Here's how the part is built. I have some questions about the finished solid (model axes, mm). A direction names the side the tool comes from. Round coordinates to 2 decimals unless told otherwise and drop trailing zeros. Order: outer loops, then holes, each group sorted by start corner. A loop starts at its lowest first (then second) coordinate and runs counter-clockwise, first axis right, second up.
Autodesk Inventor part; units mm, degrees
ref_plane "YZ Plane" through (0, 0, 0) normal (1, 0, 0) x (0, 1, 0)
ref_plane "XZ Plane" through (0, 0, 0) normal (0, 1, 0) x (-1, 0, 0)
ref_plane "XY Plane" through (0, 0, 0) normal (0, 0, 1) x (1, 0, 0)
sketch "Sketch1" plane through (0, 0, 0) normal (0, 1, 0) x (-1, 0, 0)
  line L0 (0, 9.8) -> (8.487, 4.9)
  line L1 (8.487, 4.9) -> (8.487, -4.9)
  line L2 (8.487, -4.9) -> (0, -9.8)
  line L3 (0, -9.8) -> (-8.487, -4.9)
  line L4 (-8.487, -4.9) -> (-8.487, 4.9)
  line L5 (-8.487, 4.9) -> (0, 9.8)
  point P0 (0, 0)
  point P1 (0, 0)
  dimension "d3" = 19.6
extrude "Extrusion1" add sketch "Sketch1" along normal blind 3
sketch "Sketch2" plane through (0, 3, 0) normal (0, 1, 0) x (1, 0, 0)
  circle A0 centre (0, 0) radius 5
  dimension "d4" = 10
extrude "Extrusion2" add sketch "Sketch2" along normal blind 20
fillet "Fillet1" radius 0.2 12 edges at (-4.2435, 3, 7.35) (-8.487, 3, 0) (-8.487, 0, 0) (-4.2435, 3, -7.35) (-4.2435, 0, -7.35) (4.2435, 3, -7.35) (4.2435, 0, -7.35) (8.487, 3, 0) (8.487, 0, 0) (4.2435, 3, 7.35) (4.2435, 0, 7.35) (-4.2435, 0, 7.35)
fillet "Fillet2" radius 1 1 edges at (-5, 3, 0)
properties part number "M10bolt"
1. If we section it at A-A, the plane z = 0: Write out the boundary of the cut face in (x, y).
Evaluation:
outline: (-8.49, 0.2) arc R0.2 ccw to (-8.29, 0) - (8.29, 0) arc R0.2 ccw to (8.49, 0.2) - (8.49, 2.8) arc R0.2 ccw to (8.29, 3) - (6, 3) arc R1 cw to (5, 4) - (5, 23) - (-5, 23) - (-5, 4) arc R1 cw to (-6, 3) - (-8.29, 3) arc R0.2 ccw to (-8.49, 2.8) - close
2. I need wall thicknesses on probe 1 along X at (y, z) = (11, -1); probe 2 along Y at (x, z) = (-3.5, 5); probe 3 along Z at (x, y) = (0, 17.25). Which ranges of each line are inside material? Lowest first, please.
Evaluation:
probe 1: x = -4.9 to 4.9
probe 2: y = 0 to 3
probe 3: z = -5 to 5
3. I'm going to push flat-ended pins straight in: P1, Ø8, axis at x = 6.5, y = 13, coming from the -Z side; P2, Ø6, axis at x = -6, y = 6.5, coming from the -Z side; P3, Ø5, axis at y = 9.5, z = -5, coming from the -X side. Where does each tip first touch, or does it pass through?
Evaluation:
P1: stops at z = -4.33
P2: stops at z = -4
P3: stops at x = -4.33
4. If we section it at B-B, the plane y = 7.25: Write out the boundary of the cut face in (x, z).
Evaluation:
outline: circle Ø10 at (0, 0)
5. On a 3-axis mill with a long thin cutter (end or side, diameter ignored), from which of +Z, -Z, +X, -X, +Y, -Y can I reach the whole of each face in a straight line? I mean faces 1 (the cylindrical face through (4.154, 0.057, 7.332)), 2 (the flat face through (0.1, 3, -6.2)). Say none if no direction works.
Evaluation:
face 1: +Z, +X, -Y
face 2: +Y
